The drawing under review shows one solid part. Ordinate dimensions are in mm from its lowest x, y, z. Coordinates: 2 decimals unless noted, no trailing zeros. Write each loop counter-clockwise with the first axis right and the second up, starting at its lowest first coordinate (ties: lowest second). Pieces come first, ordered by that corner, then holes.
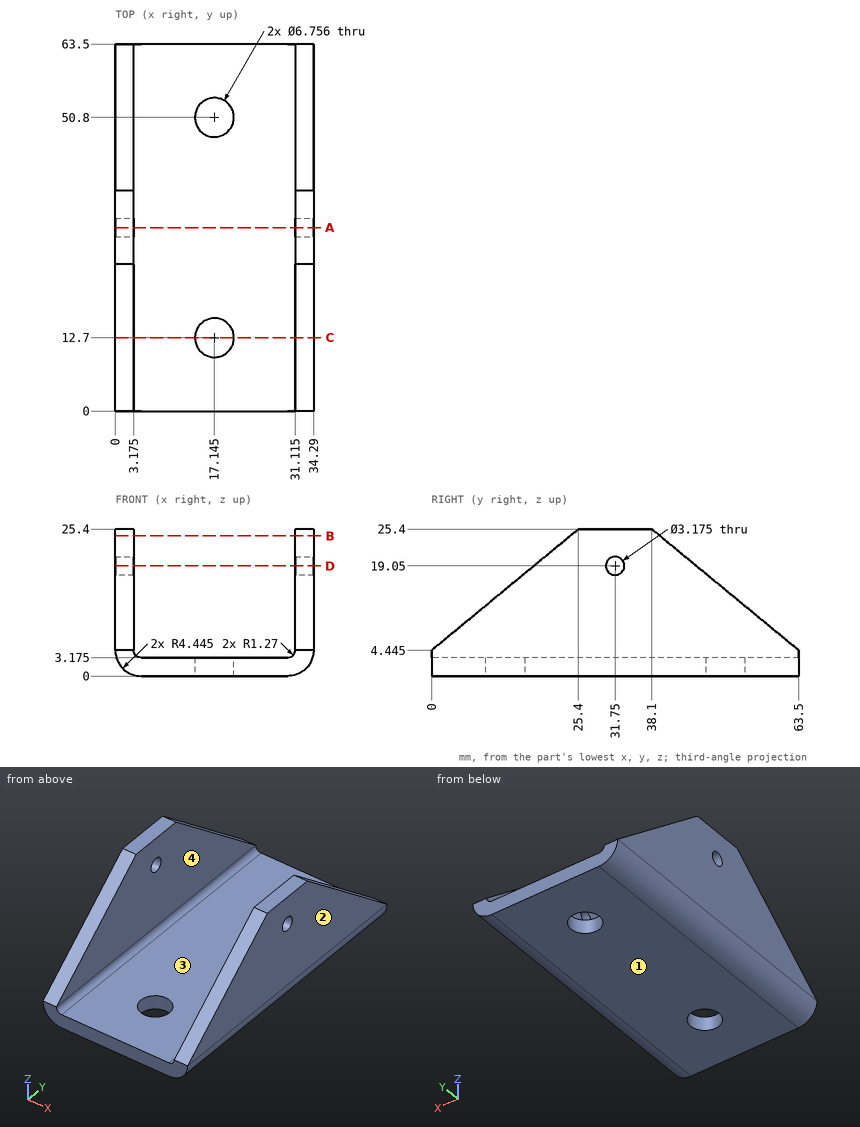
1) For L1, parallel to X at y = 24.5, z = 18.25 (1 decimal); L2, parallel to Z at x = 11, y = 53.5 (1 decimal); L3, parallel to Y at x = 2.5, z = 19.25 (1 decimal), list the stretches that pass through material, from the lowest coordinate up.
2) Consider section B-B (z = 24.25). Give the boundary of the cut face in (x, y) (1 decimal).
3) Clearance check with flat-ended pins moving along their axes: P1, Ø2, axis at y = 9, z = 15.5, coming from the +X side; P2, Ø1.5, axis at x = 30, y = 11.5, coming from the +Z side (1 decimal); P3, Ø8, axis at x = 17.145, y = 12.7, coming from the +Z side (3 decimals). State where each tip first meets the part, or that it passes through.
4) Consider section C-C (y = 12.7). Give the boundary of the cut face in (x, z) (1 decimal).
5) Consider section D-D (z = 19.05). Give the boundary of the cut face in (x, y) (1 decimal), then the cut area to 3 significant figures.
6) Consider section A-A (y = 31.75). Give the boundary of the cut face in (x, z) (1 decimal).
7) The part is to be moulded in two halves that separate along X. For the marked faces 1, 2, 3 and 4, say which applies: pulls with the +X half, pulls with the -X half, needs draft (parallel to the pull), parting line crosses it, or undercut.
Results:
1. L1: x = 0 to 3.2, 31.1 to 34.3
1. L2: z = 0 to 3.2
1. L3: y = 17.9 to 30.2, 33.3 to 45.6
2. outline: (0, 24) - (3.2, 24) - (3.2, 39.5) - (0, 39.5) - close; (31.1, 24) - (34.3, 24) - (34.3, 39.5) - (31.1, 39.5) - close
3. P1: passes through
3. P2: stops at z = 3.6
3. P3: stops at z = 3.175
4. outline: (0, 4.4) arc R4.4 ccw to (4.4, 0) - (13.8, 0) - (13.8, 3.2) - (4.4, 3.2) arc R1.3 cw to (3.2, 4.4) - (3.2, 14.9) - (0, 14.9) - close; (20.5, 0) - (29.8, 0) arc R4.4 ccw to (34.3, 4.4) - (34.3, 14.9) - (31.1, 14.9) - (31.1, 4.4) arc R1.3 cw to (29.8, 3.2) - (20.5, 3.2) - close
5. outline: (0, 17.7) - (3.2, 17.7) - (3.2, 30.2) - (0, 30.2) - close; (0, 33.3) - (3.2, 33.3) - (3.2, 45.8) - (0, 45.8) - close; (31.1, 17.7) - (34.3, 17.7) - (34.3, 30.2) - (31.1, 30.2) - close; (31.1, 33.3) - (34.3, 33.3) - (34.3, 45.8) - (31.1, 45.8) - close
5. area: 158 mm2
6. outline: (0, 4.4) arc R4.4 ccw to (4.4, 0) - (29.8, 0) arc R4.4 ccw to (34.3, 4.4) - (34.3, 17.5) - (31.1, 17.5) - (31.1, 4.4) arc R1.3 cw to (29.8, 3.2) - (4.4, 3.2) arc R1.3 cw to (3.2, 4.4) - (3.2, 17.5) - (0, 17.5) - close; (0, 20.6) - (3.2, 20.6) - (3.2, 25.4) - (0, 25.4) - close; (31.1, 20.6) - (34.3, 20.6) - (34.3, 25.4) - (31.1, 25.4) - close
7. face 1: needs draft
7. face 2: pulls with the +X half
7. face 3: undercut
7. face 4: undercut
